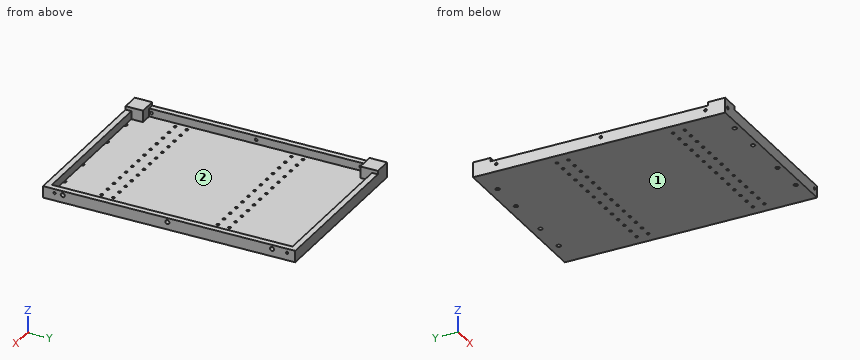
```python
from build123d import *

# Parameters (mm, degrees)
SKETCH_W        = 150
SKETCH_H        = 217
SKETCH_R        = 1.15
SKETCH_R_2      = 1.75
PAD_DEPTH       = 3
SKETCH001_W     = 150
SKETCH001_H     = 217
PAD001_DEPTH    = 7
SKETCH002_R     = 1.75
SKETCH002_R_2   = 1
POCKET_DEPTH    = 5
SKETCH003_R     = 1.15
POCKET001_DEPTH = 7.5
SKETCH004_R     = 1.15
POCKET002_DEPTH = 10
SKETCH005_W     = 15
SKETCH005_H     = 15
PAD002_DEPTH    = 3


with BuildPart() as part:
    # Sketch → Pad (new body)
    with BuildSketch(Plane.XY):
        with Locations((-75, 108.5)):
            Rectangle(SKETCH_W, SKETCH_H)
        with Locations((-140, 40)):
            Circle(SKETCH_R, mode=Mode.SUBTRACT)
        with Locations((-130, 40)):
            Circle(SKETCH_R, mode=Mode.SUBTRACT)
        with Locations((-120, 40)):
            Circle(SKETCH_R, mode=Mode.SUBTRACT)
        with Locations((-110, 40)):
            Circle(SKETCH_R, mode=Mode.SUBTRACT)
        with Locations((-100, 40)):
            Circle(SKETCH_R, mode=Mode.SUBTRACT)
        with Locations((-90, 40)):
            Circle(SKETCH_R, mode=Mode.SUBTRACT)
        with Locations((-80, 40)):
            Circle(SKETCH_R, mode=Mode.SUBTRACT)
        with Locations((-70, 40)):
            Circle(SKETCH_R, mode=Mode.SUBTRACT)
        with Locations((-60, 40)):
            Circle(SKETCH_R, mode=Mode.SUBTRACT)
        with Locations((-50, 40)):
            Circle(SKETCH_R, mode=Mode.SUBTRACT)
        with Locations((-40, 40)):
            Circle(SKETCH_R, mode=Mode.SUBTRACT)
        with Locations((-30, 40)):
            Circle(SKETCH_R, mode=Mode.SUBTRACT)
        with Locations((-20, 40)):
            Circle(SKETCH_R, mode=Mode.SUBTRACT)
        with Locations((-10, 40)):
            Circle(SKETCH_R, mode=Mode.SUBTRACT)
        with Locations((-140, 50)):
            Circle(SKETCH_R, mode=Mode.SUBTRACT)
        with Locations((-130, 50)):
            Circle(SKETCH_R, mode=Mode.SUBTRACT)
        with Locations((-120, 50)):
            Circle(SKETCH_R, mode=Mode.SUBTRACT)
        with Locations((-110, 50)):
            Circle(SKETCH_R, mode=Mode.SUBTRACT)
        with Locations((-100, 50)):
            Circle(SKETCH_R, mode=Mode.SUBTRACT)
        with Locations((-90, 50)):
            Circle(SKETCH_R, mode=Mode.SUBTRACT)
        with Locations((-80, 50)):
            Circle(SKETCH_R, mode=Mode.SUBTRACT)
        with Locations((-70, 50)):
            Circle(SKETCH_R, mode=Mode.SUBTRACT)
        with Locations((-60, 50)):
            Circle(SKETCH_R, mode=Mode.SUBTRACT)
        with Locations((-50, 50)):
            Circle(SKETCH_R, mode=Mode.SUBTRACT)
        with Locations((-40, 50)):
            Circle(SKETCH_R, mode=Mode.SUBTRACT)
        with Locations((-30, 50)):
            Circle(SKETCH_R, mode=Mode.SUBTRACT)
        with Locations((-20, 50)):
            Circle(SKETCH_R, mode=Mode.SUBTRACT)
        with Locations((-10, 50)):
            Circle(SKETCH_R, mode=Mode.SUBTRACT)
        with Locations((-140, 140)):
            Circle(SKETCH_R, mode=Mode.SUBTRACT)
        with Locations((-130, 140)):
            Circle(SKETCH_R, mode=Mode.SUBTRACT)
        with Locations((-120, 140)):
            Circle(SKETCH_R, mode=Mode.SUBTRACT)
        with Locations((-110, 140)):
            Circle(SKETCH_R, mode=Mode.SUBTRACT)
        with Locations((-100, 140)):
            Circle(SKETCH_R, mode=Mode.SUBTRACT)
        with Locations((-90, 140)):
            Circle(SKETCH_R, mode=Mode.SUBTRACT)
        with Locations((-80, 140)):
            Circle(SKETCH_R, mode=Mode.SUBTRACT)
        with Locations((-70, 140)):
            Circle(SKETCH_R, mode=Mode.SUBTRACT)
        with Locations((-60, 140)):
            Circle(SKETCH_R, mode=Mode.SUBTRACT)
        with Locations((-50, 140)):
            Circle(SKETCH_R, mode=Mode.SUBTRACT)
        with Locations((-40, 140)):
            Circle(SKETCH_R, mode=Mode.SUBTRACT)
        with Locations((-30, 140)):
            Circle(SKETCH_R, mode=Mode.SUBTRACT)
        with Locations((-20, 140)):
            Circle(SKETCH_R, mode=Mode.SUBTRACT)
        with Locations((-10, 140)):
            Circle(SKETCH_R, mode=Mode.SUBTRACT)
        with Locations((-140, 150)):
            Circle(SKETCH_R, mode=Mode.SUBTRACT)
        with Locations((-130, 150)):
            Circle(SKETCH_R, mode=Mode.SUBTRACT)
        with Locations((-120, 150)):
            Circle(SKETCH_R, mode=Mode.SUBTRACT)
        with Locations((-110, 150)):
            Circle(SKETCH_R, mode=Mode.SUBTRACT)
        with Locations((-100, 150)):
            Circle(SKETCH_R, mode=Mode.SUBTRACT)
        with Locations((-90, 150)):
            Circle(SKETCH_R, mode=Mode.SUBTRACT)
        with Locations((-80, 150)):
            Circle(SKETCH_R, mode=Mode.SUBTRACT)
        with Locations((-70, 150)):
            Circle(SKETCH_R, mode=Mode.SUBTRACT)
        with Locations((-60, 150)):
            Circle(SKETCH_R, mode=Mode.SUBTRACT)
        with Locations((-50, 150)):
            Circle(SKETCH_R, mode=Mode.SUBTRACT)
        with Locations((-40, 150)):
            Circle(SKETCH_R, mode=Mode.SUBTRACT)
        with Locations((-30, 150)):
            Circle(SKETCH_R, mode=Mode.SUBTRACT)
        with Locations((-20, 150)):
            Circle(SKETCH_R, mode=Mode.SUBTRACT)
        with Locations((-10, 150)):
            Circle(SKETCH_R, mode=Mode.SUBTRACT)
        with Locations((-125, 209)):
            Circle(SKETCH_R_2, mode=Mode.SUBTRACT)
        with Locations((-55, 209)):
            Circle(SKETCH_R_2, mode=Mode.SUBTRACT)
        with Locations((-125, 5)):
            Circle(SKETCH_R_2, mode=Mode.SUBTRACT)
        with Locations((-55, 5)):
            Circle(SKETCH_R_2, mode=Mode.SUBTRACT)
        with Locations((-25, 5)):
            Circle(SKETCH_R_2, mode=Mode.SUBTRACT)
        with Locations((-95, 5)):
            Circle(SKETCH_R_2, mode=Mode.SUBTRACT)
        with Locations((-25, 209)):
            Circle(SKETCH_R_2, mode=Mode.SUBTRACT)
        with Locations((-95, 209)):
            Circle(SKETCH_R_2, mode=Mode.SUBTRACT)
    extrude(amount=PAD_DEPTH)

    # Sketch001 → Pad001 (join)
    with BuildSketch(Plane.XY.offset(3)):
        with Locations((-75, 108.5)):
            Rectangle(SKETCH001_W, SKETCH001_H)
        Polygon((-5, 212), (-135, 212), (-135, 202), (-145, 202), (-145, 15), (-135, 15), (-135, 5), (-5, 5), align=None, mode=Mode.SUBTRACT)
    extrude(amount=PAD001_DEPTH)

    # Sketch002 → Pocket (cut)
    with BuildSketch(Plane.YZ):
        with Locations((17, 6.5)):
            Circle(SKETCH002_R)
        with Locations((107, 6.5)):
            Circle(SKETCH002_R)
        with Locations((197, 6.5)):
            Circle(SKETCH002_R)
        with Locations((10, 6.5)):
            Circle(SKETCH002_R_2)
        with Locations((210, 6.5)):
            Circle(SKETCH002_R_2)
    extrude(amount=-POCKET_DEPTH, mode=Mode.SUBTRACT)

    # Sketch003 → Pocket001 (cut, symmetric)
    with BuildSketch(Plane.YZ.offset(-150)):
        with Locations((107, 6.5)):
            Circle(SKETCH003_R)
        with Locations((17, 6.5)):
            Circle(SKETCH003_R)
        with Locations((197, 6.5)):
            Circle(SKETCH003_R)
    extrude(amount=POCKET001_DEPTH, both=True, mode=Mode.SUBTRACT)

    # Sketch004 → Pocket002 (cut)
    with BuildSketch(Plane.XZ):
        with Locations((-4, 6)):
            Circle(SKETCH004_R)
        with Locations((-146, 6)):
            Circle(SKETCH004_R)
    extrude(amount=-POCKET002_DEPTH, mode=Mode.SUBTRACT)

    # Sketch005 → Pad002 (join)
    with BuildSketch(Plane.XY.offset(10)):
        with Locations((-142.5, 209.5)):
            Rectangle(SKETCH005_W, SKETCH005_H)
        with Locations((-142.5, 7.5)):
            Rectangle(SKETCH005_W, SKETCH005_H)
    extrude(amount=PAD002_DEPTH)


solid = part.part
```
Source: CAD feature listing. Evaluate the final solid. Frame: model axes, mm. Face numbers are marked on the shaded views. Round coordinates to 2 decimals unless told otherwise and drop trailing zeros. Loops run counter-clockwise (first coordinate to the right, second up) from the corner with the lowest first, then second, coordinate; pieces in that order, holes last. Notation, with made-up numbers: M -39,89.25 L -22,89.25 A24 cw -22,119.25 Z; hole C 14.5,29.5 d5. An arc over 180 degrees is marked long. Put each result on its own line as item: value.
(1) Section B-B, the plane y = 187.5. Return loops of the section in (x, z).
Solutions:
outline: M -150,0 L 0,0 L 0,10 L -5,10 L -5,3 L -145,3 L -145,10 L -150,10 Z
(2) First-contact query: pin 1 (1.8 mm diameter, centred on x = -70, y = 140, fed in from +Z); pin 2 (4 mm diameter, centred on x = -95, y = 209, fed in from +Z). Flat tips, straight axial feed; report the tip coordinate or a pass-through.
Solutions:
pin 1: through
pin 2: z = 3
(3) Section A-A, the plane x = -84. Return loops of the section in (y, z).
Solutions:
outline: M 0,0 L 217,0 L 217,10 L 212,10 L 212,3 L 5,3 L 5,10 L 0,10 Z
(4) Pull-direction query (Y, two-part tool) for the marked faces 1 and 2; classes: released by +Y, released by -Y, zero draft, split by the parting line, or undercut.
Solutions:
face 1: zero draft
face 2: undercut
(5) Ray query, line 1 (X direction, y = 209, z = 1.05); line 2 (Y direction, x = -60, z = 2); line 3 (Y direction, x = -48, z = 5.75). Return the intervals inside material, ascending. Write a range as [from, to].
Solutions:
line 1: [-150, -126.75], [-123.25, -96.75], [-93.25, -56.75], [-53.25, -26.75], [-23.25, 0]
line 2: [0, 38.85], [41.15, 48.85], [51.15, 138.85], [141.15, 148.85], [151.15, 217]
line 3: [0, 5], [212, 217]
